```python
from build123d import *

# Parameters (mm, degrees)
BOSS_EXTRUDE1_DEPTH  = 19.05
CHAMFER1_SIZE2       = 25.4
CHAMFER1_SIZE        = 23.3906272
CHAMFER1_EDGE_2_SIZE = 25.4
HOLE2_D              = 3.175
HOLE2_DEPTH          = 31.75
HOLE2_CSINK_D        = 10.16
HOLE2_CSINK_ANGLE    = 82
HOLE2_TIP            = 0.953866233
HOLE4_D              = 3.175
HOLE4_DEPTH          = 31.75
HOLE4_CSINK_D        = 10.16
HOLE4_CSINK_ANGLE    = 82
HOLE4_TIP            = 0.953866233
HOLE5_D              = 3.175
HOLE5_DEPTH          = 38.1
HOLE5_CSINK_D        = 10.16
HOLE5_CSINK_ANGLE    = 82
HOLE5_TIP            = 0.953866233
HOLE6_D              = 3.175
HOLE6_DEPTH          = 38.1
HOLE6_CSINK_D        = 10.16
HOLE6_CSINK_ANGLE    = 82
HOLE6_TIP            = 0.953866233


with BuildPart() as part:
    # Sketch1 → Boss-Extrude1 (new body)
    with BuildSketch(Plane.XY):
        with BuildLine():
            Line((12.7, 12.7), (12.7, -415.185594934))
            ThreePointArc((12.7, -415.185594934), (27.339445595, -436.32629993), (2.687239133, -443.641454859))
            Line((2.687239133, -443.641454859), (-518.461959982, -601.369999539))
            Line((-518.461959982, -601.369999539), (-477.533889468, -736.6))
            Line((-477.533889468, -736.6), (103.700681611, -560.686301639))
            Line((103.700681611, -560.686301639), (155.492294041, 12.7))
            Line((155.492294041, 12.7), (12.7, 12.7))
        make_face()
    extrude(amount=-BOSS_EXTRUDE1_DEPTH)

    # Chamfer1
    chamfer1_edges = [part.edges().sort_by_distance(p)[0] for p in [
        (155.492294041, 12.7, -9.525),
    ]]
    chamfer(chamfer1_edges, length=CHAMFER1_SIZE, length2=CHAMFER1_SIZE2)

    # Chamfer1 edge 2
    chamfer1_edge_2_edges = [part.edges().sort_by_distance(p)[0] for p in [
        (-477.533889468, -736.6, -9.525),
    ]]
    chamfer(chamfer1_edge_2_edges, length=CHAMFER1_EDGE_2_SIZE)

    # Hole2
    with Locations(Plane(origin=(0, 10.424290059, 165.474999994), x_dir=(0, 0, -1), z_dir=(-1, 0, 0))):
        with Locations((-155.949999994, 107.734820482), (155.949999994, 107.734820482), (155.949999994, 327.755881328), (174.999999994, 85.732714397), (174.999999994, 349.757987412), (-174.999999994, 349.757987412), (-174.999999994, 85.732714397), (-155.949999994, 327.755881328)):
            CounterSinkHole(HOLE2_D / 2, HOLE2_CSINK_D / 2, depth=HOLE2_DEPTH, counter_sink_angle=HOLE2_CSINK_ANGLE)
            with Locations((0, 0, -(HOLE2_DEPTH + HOLE2_TIP / 2))):  # 118° drill point
                Cone(0, HOLE2_D / 2, HOLE2_TIP, mode=Mode.SUBTRACT)

    # Hole4
    with Locations(Plane(origin=(264.696145853, -351.07416346, 165.474999994), x_dir=(0, 0, -1), z_dir=(-0.289678603, 0.957123977, 0))):
        with Locations((174.999999994, 685.961004241), (174.999999994, 549.837259632), (174.999999994, 413.713515022), (81.549999997, 779.649723129), (81.549999997, 652.344645962), (62.499999997, 662.953402392), (62.499999997, 769.040966698), (-62.499999997, 769.040966698), (-62.499999997, 662.953402392), (-81.549999997, 652.344645962), (-81.549999997, 779.649723129), (-174.999999994, 413.713515022), (-174.999999994, 549.837259632), (-174.999999994, 685.961004241), (-82.737499997, 600.384620239), (0, 600.384620239), (82.737499997, 600.384620239), (0, 376.737770337), (-82.737499997, 376.737770337), (82.737499997, 376.737770337)):
            CounterSinkHole(HOLE4_D / 2, HOLE4_CSINK_D / 2, depth=HOLE4_DEPTH, counter_sink_angle=HOLE4_CSINK_ANGLE)
            with Locations((0, 0, -(HOLE4_DEPTH + HOLE4_TIP / 2))):  # 118° drill point
                Cone(0, HOLE4_D / 2, HOLE4_TIP, mode=Mode.SUBTRACT)

    # Hole5
    with Locations(Plane(origin=(155.286738577, 10.424290059, -19.05), x_dir=(-0.089959629, -0.995945413, 0), z_dir=(0, 0, -1))):
        with Locations((46.221112845, 113.488854888), (39.39759596, 37.945520226), (412.28786892, 80.423559293), (407.308516105, 25.297013484), (513.561319184, 161.164706775), (597.46020397, 127.267357003), (610.543339245, 159.649253123), (694.322923815, 367.011001477), (526.644454459, 193.546602895), (610.424039029, 400.908351249)):
            CounterSinkHole(HOLE5_D / 2, HOLE5_CSINK_D / 2, depth=HOLE5_DEPTH, counter_sink_angle=HOLE5_CSINK_ANGLE)
            with Locations((0, 0, -(HOLE5_DEPTH + HOLE5_TIP / 2))):  # 118° drill point
                Cone(0, HOLE5_D / 2, HOLE5_TIP, mode=Mode.SUBTRACT)

    # Hole6
    with Locations(Plane(origin=(-643.705760022, -231.394989772, 165.474999994), x_dir=(0, 0, -1), z_dir=(-0.957123977, -0.289678603, 0))):
        with Locations((-108.649999997, 332.89193461), (108.649999997, 332.89193461), (207.774999994, 332.89193461), (174.999999994, 448.336332751), (135.266666663, 384.042401694), (176.283333328, 384.042401694), (-174.999999994, 448.336332751), (-135.266666663, 384.042401694), (-176.283333328, 384.042401694), (-207.774999994, 332.89193461)):
            CounterSinkHole(HOLE6_D / 2, HOLE6_CSINK_D / 2, depth=HOLE6_DEPTH, counter_sink_angle=HOLE6_CSINK_ANGLE)
            with Locations((0, 0, -(HOLE6_DEPTH + HOLE6_TIP / 2))):  # 118° drill point
                Cone(0, HOLE6_D / 2, HOLE6_TIP, mode=Mode.SUBTRACT)


solid = part.part
```
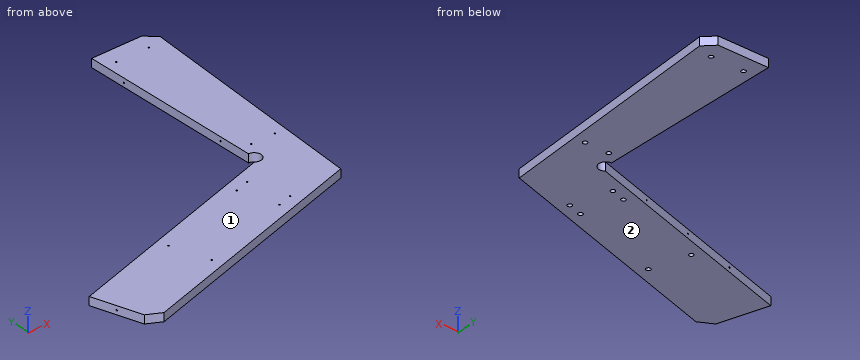
CAD build for the part. Positions are in the model's coordinates, mm. Face numbers are marked on the shaded views. Round coordinates to 2 decimals unless told otherwise and drop trailing zeros. Loops run counter-clockwise (first coordinate to the right, second up) from the corner with the lowest first, then second, coordinate; pieces in that order, holes last. Notation, with made-up numbers: M 26,-15.5 L 45,-15.5 A17 ccw 45,2.5 Z; hole C 29,85.5 d11. An arc over 180 degrees is marked long. Return JSON: item names as keys, results as strings. Group by question number.
(1) Saw through at A-A, the plane z = -4.5. Give the number of separate pieces and of enclosed holes in the cut face, and give its area (3 significant figures).
(2) Wall check: probe 1 along X at (y, z) = (-25.4, -9.75); probe 2 along X at (y, z) = (-25, -4.5); probe 3 along Y at (x, z) = (-347, -4.5). Give the ranges that are in metal, low to high. Write a range as [from, to].
(3) Saw through at C-C, the plane y = -221. List the corners of the cut face in (x, z), and give its area (3 significant figures).
(4) Drop flat-ended pins along their axis: P1, Ø4, axis at x = -58.64, y = -583.28, coming from the +Z side; P2, Ø1.5, axis at y = -373.5, z = -13.5, coming from the -X side; P3, Ø2, axis at x = 74.5, z = -16.5, coming from the -Y side; P4, Ø3.5, axis at x = 93.45, y = -392.96, coming from the -Z side. Give the stop position or say it passes through.
(5) Mould opens along Z. For the marked faces 1 and 2 say: +Z half, -Z half, draft (parallel to the pull), parting line (faces both ways), or undercut.
(6) Saw through at B-B, the plane x = -100. List the corners of the cut face in (y, z).
Answer list:
{
 "1": {"separate pieces": "1", "enclosed holes": "10", "area": "143,000 mm2"},
 "2": {"probe 1": "[12.7, 36.51], [39.69, 112.36], [115.54, 152.05]", "probe 2": "[12.7, 36.56], [39.64, 112.41], [115.49, 152.09]", "probe 3": "[-697.09, -549.48]"},
 "3": {"outline": "M 12.7,-19.05 L 134.38,-19.05 L 134.38,0 L 12.7,0 Z", "area": "2,320 mm2"},
 "4": {"P1": "z = 0", "P2": "x = 12.7", "P3": "y = -569.83", "P4": "z = -15.22"},
 "5": {"face 1": "+Z half", "face 2": "-Z half"},
 "6": {"outline": "M -622.34,-19.05 L -474.72,-19.05 L -474.72,0 L -622.34,0 Z"}
}
